Geometry check sheet. Reference: the model listing, model coordinates, mm. Face numbers are marked on the shaded views. A direction names the side the tool comes from. Coordinates: 2 decimals unless noted, no trailing zeros. Loops run counter-clockwise (first coordinate to the right, second up) from the corner with the lowest first, then second, coordinate; pieces in that order, holes last. Notation, with made-up numbers: (47.5, 66.25) - (65.5, 66.25) arc R15 cw to (65.5, 83.25) - close; hole circle Ø11 at (8.25, 27). An arc over 180 degrees is marked (long way). Write each question's results on one line, items separated by ' | '. Start each with the question number.
(1) Sectioned sample at D-D (y = 102). Enter the section's corners in (x, z).
(2) Material ranges on probe 1 along Y at (x, z) = (11, -15.5); probe 2 along X at (y, z) = (74, 0); probe 3 along Z at (x, y) = (-0.5, 12.5), recorded low to high.
(3) Sectioned sample at B-B (x = 0). Enter the section's corners in (y, z).
(4) Go/stop test with flat-tipped pins: pin 1 Ø5 at (x, y) = (-1.5, 18.5) entering from +Z; pin 2 Ø10 at (x, z) = (16.5, 16) entering from -Y; pin 3 Ø3 at (x, y) = (11, 50) entering from +Z; pin 4 Ø1.5 at (y, z) = (28, -3) entering from -X. Record where each tip stops, or that it passes through.
(5) Access from +Z, -Z, +X, -X, +Y, -Y to the whole of each face (thin tool, end or side, straight path). Record for the marked faces 1 and 2.
(6) Sectioned sample at C-C (y = 77.5). Enter the section's corners in (x, z).
(7) Sectioned sample at A-A (z = 0). Enter the section's corners in (x, y).
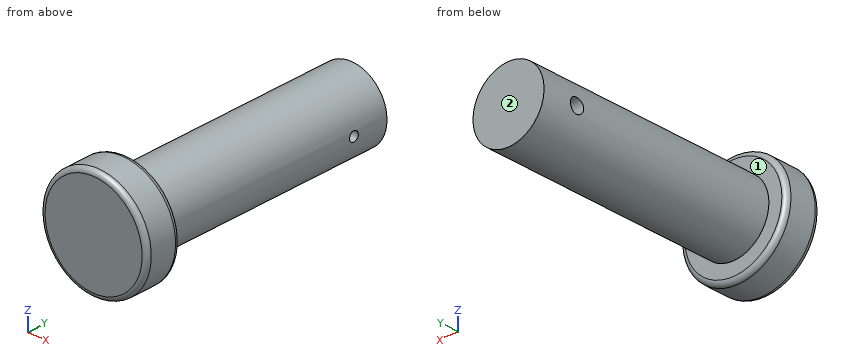
Autodesk Inventor part; units mm, degrees
ref_plane "YZ Plane" through (0, 0, 0) normal (1, 0, 0) x (0, 1, 0)
ref_plane "XZ Plane" through (0, 0, 0) normal (0, 1, 0) x (-1, 0, 0)
ref_plane "XY Plane" through (0, 0, 0) normal (0, 0, 1) x (1, 0, 0)
sketch "Sketch1" plane through (0, 0, 0) normal (0, 1, 0) x (-1, 0, 0)
  circle A0 centre (0, 0) radius 22.5
  dimension "d0" = 45
extrude "Extrusion1" add sketch "Sketch1" along normal blind 15
sketch "Sketch2" plane through (0, 15, 0) normal (0, 1, 0) x (1, 0, 0)
  circle A0 centre (0, 0) radius 15
  dimension "d3" = 30
extrude "Extrusion2" add sketch "Sketch2" along normal blind 102
sketch "Sketch3" plane through (0, 0, 0) normal (0, 0, 1) x (1, 0, 0)
  line L0 (-15, 15) -> (-15, 117)
  line L1 (-15, 102) -> (15, 102)
  line L2 (15, 15) -> (15, 117)
  line L3 (15, 117) -> (-15, 117)
  line L4 (-15, 102) -> (-15, 105)
  line L5 (15, 102) -> (15, 104)
  line L6 (15, 104) -> (-15, 105)
  point P0 (0, 0)
  dimension "d6" = 15
  dimension "d7" = 3
  dimension "d8" = 2
revolve "Revolution1" cut sketch "Sketch3" angle 360 about axis through (-15, 102, 0) along (1, 0, 0) contours L0 L6 L2 L1
fillet "Fillet1" radius 2 2 edges at (22.5, 15, 0) (22.5, 0, 0)
properties part number "pin"
Outcome:
1) outline: (-14.7, -2.99) arc R15 ccw to (14.87, -2) - close; (-14.7, 2.99) - (14.87, 2) arc R15 ccw to start
2) probe 1: y = 0 to 15 | probe 2: x = -15 to 15 | probe 3: z = -22.49 to 22.49
3) outline: (0, -20.5) arc R2 ccw to (2, -22.5) - (13, -22.5) arc R2 ccw to (15, -20.5) - (15, -15) - (117, -15) - (117, 15) - (15, 15) - (15, 20.5) arc R2 ccw to (13, 22.5) - (2, 22.5) arc R2 ccw to (0, 20.5) - close; hole circle Ø5 at (102, 0)
4) pin 1: stops at z = 15 | pin 2: stops at y = 0 | pin 3: stops at z = 11.61 | pin 4: stops at x = -14.83
5) face 1: +Y | face 2: +Z, -Z, +X, -X, +Y
6) outline: circle Ø30 at (0, 0)
7) outline: (-22.5, 2) arc R2 ccw to (-20.5, 0) - (20.5, 0) arc R2 ccw to (22.5, 2) - (22.5, 13) arc R2 ccw to (20.5, 15) - (15, 15) - (15, 100) - (-15, 99) - (-15, 15) - (-20.5, 15) arc R2 ccw to (-22.5, 13) - close; (-15, 105) - (15, 104) - (15, 117) - (-15, 117) - close
